Design review of the part built by this model. Coordinates are the model's own, in mm. Face numbers are marked on the shaded views. Round coordinates to 2 decimals unless told otherwise and drop trailing zeros. Loops run counter-clockwise (first coordinate to the right, second up) from the corner with the lowest first, then second, coordinate; pieces in that order, holes last. Notation, with made-up numbers: M 31.5,-18.75 L 59.5,-18.75 A35 ccw 59.5,16.25 Z; hole C 89,17 d8. An arc over 180 degrees is marked long. One line per item, written item: value. Start each with the question number.
Item 1: We need section C-C (x = 2.5). Write out the cut boundary in (y, z).
Item 2: We need section D-D (x = 9.5). Write out the cut boundary in (y, z), then the cut area to 3 significant figures.
Item 3: Mouldability with a two-part tool opening along Z and no side actions: class the marked faces 1, 2 and 3 as released by +Z, released by -Z, zero draft, split by the parting line, or undercut.
Item 4: We need section A-A (y = 5). Write out the cut boundary in (x, z), then the cut area to 3 significant figures.
Item 5: We need section B-B (z = 13). Write out the cut boundary in (x, y).
Item 6: For line 1 along X through (y, z) = (4, 2.5); line 2 along Z through (x, y) = (13.25, 5.75); line 3 along Z through (x, y) = (3.25, 2.75), list the stretches that pass through material, from the lowest coordinate up.
from build123d import *

# Parameters (mm, degrees)
SKETCH1_W           = 15
SKETCH1_H           = 15
BOSS_EXTRUDE1_DEPTH = 7
SKETCH3_R           = 1
CUT_EXTRUDE1_DEPTH  = 23.338307904
FILLET1_R           = 3


with BuildPart() as part:
    # Sketch1 → Boss-Extrude1 (new body)
    with BuildSketch(Plane(origin=(0, 0, 0), x_dir=(1, 0, 0), z_dir=(0, 1, 0))):
        with Locations((7.5, -7.5)):
            Rectangle(SKETCH1_W, SKETCH1_H)
    extrude(amount=BOSS_EXTRUDE1_DEPTH)

    # Sketch2 → Cut-Revolve1 (revolve, cut)
    with BuildSketch(Plane(origin=(0, 7, 0), x_dir=(1, 0, 0), z_dir=(0, 1, 0))):
        with BuildLine():
            Line((12.7, -7.5), (2.3, -7.5))
            ThreePointArc((2.3, -7.5), (7.5, -12.7), (12.7, -7.5))
        make_face()
    revolve(axis=Axis((12.7, 7, 7.5), (-1, 0, 0)), mode=Mode.SUBTRACT)

    # Sketch3 → Cut-Extrude1 (cut, through all)
    with BuildSketch(Plane(origin=(0, 7, 0), x_dir=(1, 0, 0), z_dir=(0, 1, 0))):
        with Locations(Location((2.5, -12.5, 0), (0, 0, 270))):
            Circle(SKETCH3_R)
        with Locations(Location((12.5, -12.5, 0), (0, 0, 270))):
            Circle(SKETCH3_R)
        with Locations(Location((12.5, -2.5, 0), (0, 0, 270))):
            Circle(SKETCH3_R)
        with Locations(Location((2.5, -2.5, 0), (0, 0, 270))):
            Circle(SKETCH3_R)
    extrude(amount=-CUT_EXTRUDE1_DEPTH, mode=Mode.SUBTRACT)

    # Fillet1
    fillet1_edges = [part.edges().sort_by_distance(p)[0] for p in [
        (0, 3.5, 0),
        (15, 3.5, 0),
        (15, 3.5, 15),
        (0, 3.5, 15),
    ]]
    fillet(fillet1_edges, radius=FILLET1_R)


solid = part.part
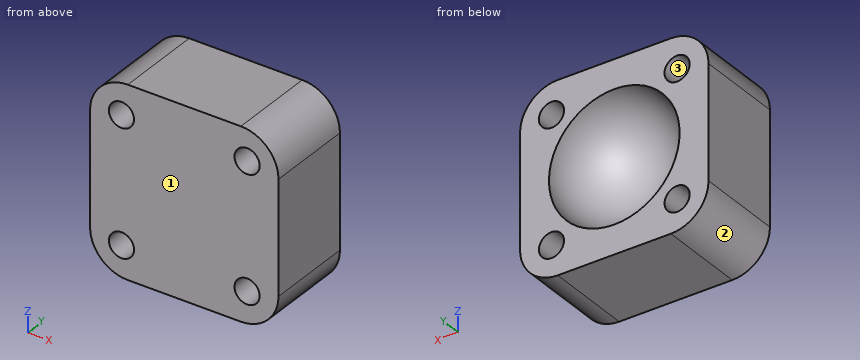
A:
1. outline: M 0,0.04 L 7,0.04 L 7,1.5 L 0,1.5 Z; M 0,3.5 L 7,3.5 L 7,6.07 A1.43 cw 7,8.93 L 7,11.5 L 0,11.5 Z; M 0,13.5 L 7,13.5 L 7,14.96 L 0,14.96 Z
2. outline: M 0,0 L 7,0 L 7,2.7 A4.8 cw 7,12.3 L 7,15 L 0,15 Z
2. area: 68.8 mm2
3. face 1: zero draft
3. face 2: released by -Z
3. face 3: undercut
4. outline: M 0,3 A3 ccw 3,0 L 12,0 A3 ccw 15,3 L 15,12 A3 ccw 12,15 L 3,15 A3 ccw 0,12 Z; hole C 2.5,2.5 d2; hole C 2.5,12.5 d2; hole C 7.5,7.5 d9.6; hole C 12.5,2.5 d2; hole C 12.5,12.5 d2
4. area: 132 mm2
5. outline: M 0.17,0 L 1.63,0 L 1.63,7 L 0.17,7 Z; M 3.37,0 L 11.63,0 L 11.63,7 L 3.37,7 Z; M 13.37,0 L 14.83,0 L 14.83,7 L 13.37,7 Z
6. line 1: 0.04 to 1.5, 3.5 to 11.5, 13.5 to 14.96
6. line 2: 0.27 to 1.84, 3.16 to 11.84, 13.16 to 14.73
6. line 3: 0 to 1.84, 3.16 to 11.84, 13.16 to 15
